Verification items for the finished model (mm, model axes). A direction names the side the tool comes from. Round coordinates to 2 decimals unless told otherwise and drop trailing zeros. Write each loop counter-clockwise with the first axis right and the second up, starting at its lowest first coordinate (ties: lowest second). Pieces come first, ordered by that corner, then holes. Notation, with made-up numbers: M 45.5,77 L 74.5,77 A24 ccw 74.5,113 Z; hole C -16,-12.75 d1. An arc over 180 degrees is marked long. One line per item, written item: value. Start each with the question number.
Item 1: Gauge pin test, flat ends, axial feed: pin 1 (17 mm diameter, centred on x = 90.5, y = -90.5, fed in from -Z); pin 2 (2.5 mm diameter, centred on x = -115, y = -80, fed in from +Z); pin 3 (22.5 mm diameter, centred on y = -73, z = -188, fed in from +X). Record the tip position at first contact, or that the pin passes through.
Item 2: Draft check along Z on faces 6 (the face through (88, -63, -150)), 7 (the face through (125, -87.3, 236.6)), 8 (the face through (-2, 21, -300)), 9 (the face through (74, -77, -248)). Enter one of: +Z half, -Z half, draft (parallel to the pull), parting line (faces both ways), or undercut.
Item 3: Tool access check on faces 1 (the face through (-88, -63, 150)), 2 (the face through (74, -88, 260)), 3 (the face through (-88, -25, 226)), 4 (the face through (74, -88, -237)), 5 (the face through (-74, -88, 258)). Record the directions out of +Z, -Z, +X, -X, +Y, -Y that give a thin tool (end or side, any length) a straight path to the whole face; none if there is none.
Item 4: Thickness scan on probe 1 along Y at (x, z) = (105, 259.2); probe 2 along Z at (x, y) = (40, -70.5); probe 3 along Y at (x, z) = (51, -155). Record the ranges inside material, lowest first. Write a range as from..to.
Item 5: Section check A-A, the plane x = -86. Record the cut outline in (y, z).
Item 6: Section check B-B, the plane y = -35. Record the cut outline in (x, z), then the cut area to 3 significant figures.
Item 7: Section check C-C, the plane z = 173. Record the cut outline in (x, y).
from build123d import *

# Parameters (mm, degrees)
BOSS_EXTRUDE1_DEPTH       = 150
BOSS_EXTRUDE1_DEPTH_BACK  = 150
SKETCH2_W                 = 600
SKETCH2_H                 = 200
SKETCH3_W                 = 150
SKETCH3_H                 = 75
CUT_EXTRUDE1_DEPTH        = 125
SKETCH4_W                 = 25
SKETCH4_H                 = 25
SKETCH4_W_2               = 21
SKETCH4_H_2               = 21
BOSS_EXTRUDE2_DEPTH       = 100
SKETCH5_R                 = 2
CUT_EXTRUDE2_DEPTH        = 25
MIRROR3_COPY_1_SKETCH_W   = 25
MIRROR3_COPY_1_SKETCH_H   = 25
MIRROR3_COPY_1_SKETCH_W_2 = 21
MIRROR3_COPY_1_SKETCH_H_2 = 21
MIRROR3_COPY_1_DEPTH      = 100
MIRROR3_COPY_2_SKETCH_R   = 2
MIRROR3_COPY_2_DEPTH      = 25


with BuildPart() as part:
    # Sketch2 → Boss-Extrude1 (new, two sides: drawn at the far end of the back side and taken through both)
    with BuildSketch(Plane(origin=(0, 0, 0), x_dir=(0, 0, -1), z_dir=(1, 0, 0)).offset(-BOSS_EXTRUDE1_DEPTH_BACK)):
        Rectangle(SKETCH2_W, SKETCH2_H)
    extrude(amount=BOSS_EXTRUDE1_DEPTH + BOSS_EXTRUDE1_DEPTH_BACK)

    # Sketch3 → Cut-Extrude1 (cut)
    with BuildSketch(Plane(origin=(150, 0, 0), x_dir=(0, 0, -1), z_dir=(1, 0, 0))):
        with Locations((-225, -62.5)):
            Rectangle(SKETCH3_W, SKETCH3_H)
        with Locations((225, -62.5)):
            Rectangle(SKETCH3_W, SKETCH3_H)
    cut_extrude1 = extrude(amount=-CUT_EXTRUDE1_DEPTH, mode=Mode.SUBTRACT)

    # Mirror1: Cut-Extrude1 across plane
    add(cut_extrude1.mirror(Plane(origin=(0, 0, 0), x_dir=(0, 0, 1), z_dir=(1, 0, 0))), mode=Mode.SUBTRACT)

    # Sketch4 → Boss-Extrude2 (add)
    with BuildSketch(Plane(origin=(25, 0, 0), x_dir=(0, 0, -1), z_dir=(1, 0, 0))):
        with Locations((-247.5, -87.5)):
            Rectangle(SKETCH4_W, SKETCH4_H)
        with Locations((-247.5, -87.5)):
            Rectangle(SKETCH4_W_2, SKETCH4_H_2, mode=Mode.SUBTRACT)
    boss_extrude2 = extrude(amount=BOSS_EXTRUDE2_DEPTH)

    # Sketch5 → Cut-Extrude2 (cut)
    with BuildSketch(Plane.XY.offset(260)):
        with Locations((115, -80)):
            Circle(SKETCH5_R)
        with Locations((105, -80)):
            Circle(SKETCH5_R)
        with Locations((95, -80)):
            Circle(SKETCH5_R)
        with Locations((115, -95)):
            Circle(SKETCH5_R)
        with Locations((105, -95)):
            Circle(SKETCH5_R)
        with Locations((95, -95)):
            Circle(SKETCH5_R)
    cut_extrude2 = extrude(amount=-CUT_EXTRUDE2_DEPTH, mode=Mode.SUBTRACT)

    # Mirror2: Boss-Extrude2, Cut-Extrude2 across plane
    add(boss_extrude2.mirror(Plane(origin=(0, 0, 0), x_dir=(0, 0, 1), z_dir=(1, 0, 0))))
    add(cut_extrude2.mirror(Plane(origin=(0, 0, 0), x_dir=(0, 0, 1), z_dir=(1, 0, 0))), mode=Mode.SUBTRACT)

    # Mirror3: Boss-Extrude2, Cut-Extrude2 across plane
    add(boss_extrude2.mirror(Plane.XY))
    add(cut_extrude2.mirror(Plane.XY), mode=Mode.SUBTRACT)

    # Mirror3 copy 1 sketch → Mirror3 copy 1 (add)
    with BuildSketch(Plane.ZY.offset(25)):
        with Locations((-247.5, -87.5)):
            Rectangle(MIRROR3_COPY_1_SKETCH_W, MIRROR3_COPY_1_SKETCH_H)
        with Locations((-247.5, -87.5)):
            Rectangle(MIRROR3_COPY_1_SKETCH_W_2, MIRROR3_COPY_1_SKETCH_H_2, mode=Mode.SUBTRACT)
    extrude(amount=MIRROR3_COPY_1_DEPTH)

    # Mirror3 copy 2 sketch → Mirror3 copy 2 (cut)
    with BuildSketch(Plane(origin=(0, 0, -260), x_dir=(-1, 0, 0), z_dir=(0, 0, -1))):
        with Locations((115, -80)):
            Circle(MIRROR3_COPY_2_SKETCH_R)
        with Locations((105, -80)):
            Circle(MIRROR3_COPY_2_SKETCH_R)
        with Locations((95, -80)):
            Circle(MIRROR3_COPY_2_SKETCH_R)
        with Locations((115, -95)):
            Circle(MIRROR3_COPY_2_SKETCH_R)
        with Locations((105, -95)):
            Circle(MIRROR3_COPY_2_SKETCH_R)
        with Locations((95, -95)):
            Circle(MIRROR3_COPY_2_SKETCH_R)
    extrude(amount=-MIRROR3_COPY_2_DEPTH, mode=Mode.SUBTRACT)


solid = part.part
Response values:
1. pin 1: stops at z = -260
1. pin 2: stops at z = 150
1. pin 3: stops at x = 25
2. face 6: undercut
2. face 7: draft
2. face 8: -Z half
2. face 9: undercut
3. face 1: -X, -Y
3. face 2: +Z, +X, -Y
3. face 3: +Z, -X
3. face 4: +X
3. face 5: -X
4. probe 1: y = -100..-97, -93..-82, -78..-75, -25..100
4. probe 2: z = -150..150
4. probe 3: y = -25..100
5. outline: M -100,-260 L -75,-260 L -75,-235 L -100,-235 Z; M -100,-150 L -25,-150 L -25,-300 L 100,-300 L 100,300 L -25,300 L -25,150 L -100,150 Z; M -100,235 L -75,235 L -75,260 L -100,260 Z; hole M -98,-258 L -77,-258 L -77,-237 L -98,-237 Z; hole M -98,237 L -77,237 L -77,258 L -98,258 Z
6. outline: M -150,-150 L -25,-150 L -25,-300 L 25,-300 L 25,-150 L 150,-150 L 150,150 L 25,150 L 25,300 L -25,300 L -25,150 L -150,150 Z
6. area: 105,000 mm2
7. outline: M -150,-25 L -25,-25 L -25,-100 L 25,-100 L 25,-25 L 150,-25 L 150,100 L -150,100 Z
